Here's how the part is built. I have some questions about the finished solid (model axes, mm). A direction names the side the tool comes from. Coordinates: 2 decimals unless noted, no trailing zeros. Write each loop counter-clockwise with the first axis right and the second up, starting at its lowest first coordinate (ties: lowest second). Pieces come first, ordered by that corner, then holes. Notation, with made-up numbers: (62, 51.25) -> (116, 51.25) arc R22 ccw to (116, 81.25) -> close; hole circle Ø7 at (-11.5, 21.5). An arc over 180 degrees is marked (long way). Use CSV: the item, a comma, the result in double quotes. Start each with the question number.
```python
from build123d import *

# Parameters (mm, degrees)
SKETCH1_R           = 50
BOSS_EXTRUDE1_DEPTH = 10
SKETCH2_R           = 2.5
SKETCH2_W           = 5
SKETCH2_H           = 25
SKETCH2_W_2         = 25
SKETCH2_H_2         = 5
CUT_EXTRUDE1_DEPTH  = 11


with BuildPart() as part:
    # Sketch1 → Boss-Extrude1 (new body)
    with BuildSketch(Plane(origin=(0, 0, 0), x_dir=(1, 0, 0), z_dir=(0, 1, 0))):
        Circle(SKETCH1_R)
    extrude(amount=BOSS_EXTRUDE1_DEPTH)

    # Sketch2 → Cut-Extrude1 (cut, through all)
    with BuildSketch(Plane(origin=(0, 10, 0), x_dir=(1, 0, 0), z_dir=(0, 1, 0))):
        Circle(SKETCH2_R)
        with Locations((-20, 0)):
            Rectangle(SKETCH2_W, SKETCH2_H)
        with Locations((0, -20)):
            Rectangle(SKETCH2_W_2, SKETCH2_H_2)
    extrude(amount=-CUT_EXTRUDE1_DEPTH, mode=Mode.SUBTRACT)


solid = part.part
```
Item 1: If I drill on line 1 along Z through (x, y) = (0, 3.25); line 2 along X through (y, z) = (8.25, 0); line 3 along Z through (x, y) = (-6, 8.25), over which ranges is the centre line in solid material (lowest first)?
Item 2: I want a section at C-C on y = 3.75. Please give me the cut outline in (x, z).
Item 3: Thinking about a two-plate mould opening in X: for faces 3 (the flat face through (10, 0, -1)), 4 (the cylindrical face through (47.69, 4.93, -15.02)), 5 (the cylindrical face through (-0.54, 5.07, 2.44)), which applies, +X half, -X half, draft (parallel to the pull), parting line (faces both ways), or undercut?
Item 4: I want a section at D-D on z = 14. Please give me the cut outline in (x, y).
Item 5: I'm going to push flat-ended pins straight in: pin 1 (1.5 mm diameter, centred on x = -19.5, y = 4.5, fed in from +Z); pin 2 (2.5 mm diameter, centred on y = 7, z = 19, fed in from +X); pin 3 (3 mm diameter, centred on x = 11.5, z = -35, fed in from -Y); pin 4 (6 mm diameter, centred on x = -4, y = 3, fed in from -Z). Where does each tip first touch, or does it pass through?
Item 6: I want a section at B-B on z = 0. Please give me the cut outline in (x, y).
Item 7: Which directions (+Z, -Z, +X, -X, +Y, -Y) give clear straight access to the entire face, cutting with the end or side of a thin tool? Please do faces 1 (the flat face through (-22.5, 5, 0)), 2 (the flat face through (10, 10, -1)).
Item 8: I want a section at A-A on x = 0. Please give me the cut outline in (y, z), then the cut area to 3 significant figures.
Geometry says:
1,line 1,"-50 to -2.5, 2.5 to 17.5, 22.5 to 50"
1,line 2,"-50 to -22.5, -17.5 to -2.5, 2.5 to 50"
1,line 3,"-49.64 to 17.5, 22.5 to 49.64"
2,outline,"circle Ø100 at (0, 0); hole (-22.5, -12.5) -> (-17.5, -12.5) -> (-17.5, 12.5) -> (-22.5, 12.5) -> close; hole (-12.5, 17.5) -> (12.5, 17.5) -> (12.5, 22.5) -> (-12.5, 22.5) -> close; hole circle Ø5 at (0, 0)"
3,face 3,"draft"
3,face 4,"parting line"
3,face 5,"undercut"
4,outline,"(-48, 0) -> (48, 0) -> (48, 10) -> (-48, 10) -> close"
5,pin 1,"z = 46.35"
5,pin 2,"x = 46.74"
5,pin 3,"y = 0"
5,pin 4,"z = -49.99"
6,outline,"(-50, 0) -> (-22.5, 0) -> (-22.5, 10) -> (-50, 10) -> close; (-17.5, 0) -> (-2.5, 0) -> (-2.5, 10) -> (-17.5, 10) -> close; (2.5, 0) -> (50, 0) -> (50, 10) -> (2.5, 10) -> close"
7,face 1,"+Y, -Y"
7,face 2,"+Z, -Z, +X, -X, +Y"
8,outline,"(0, -50) -> (10, -50) -> (10, -2.5) -> (0, -2.5) -> close; (0, 2.5) -> (10, 2.5) -> (10, 17.5) -> (0, 17.5) -> close; (0, 22.5) -> (10, 22.5) -> (10, 50) -> (0, 50) -> close"
8,area,"900 mm2"
